Autodesk Inventor part; units mm, degrees
ref_plane "YZ Plane" through (0, 0, 0) normal (1, 0, 0) x (0, 1, 0)
ref_plane "XZ Plane" through (0, 0, 0) normal (0, 1, 0) x (-1, 0, 0)
ref_plane "XY Plane" through (0, 0, 0) normal (0, 0, 1) x (1, 0, 0)
sketch "Sketch1" plane through (0, 0, 0) normal (0, 0, 1) x (1, 0, 0)
  circle A0 centre (0, 0) radius 65
  dimension "d0" = 130
extrude "Extrusion1" add sketch "Sketch1" along normal blind 1.5
sketch "Sketch2" plane through (0, 0, 1.5) normal (0, 0, 1) x (1, 0, 0)
  circle A0 centre (0, 0) radius 57 construction
  point P0 (-57, 0)
  dimension "d3" = 114
hole "Hole1" at (-57, 0, 1.5) direction (0, 0, -1) diameter 7 end through all
pattern_circular "Circular Pattern1" count 8 over 360 about axis through (0, 0, -10) along (0, 0, 1) of "Hole1"
properties material "Rubber"
Part model, mm, in its own coordinate system. Give positions to 0.01 mm unless a question says otherwise; leave off trailing zeros. Order: outer loops, then holes, each group sorted by start corner. A loop starts at its lowest first (then second) coordinate and runs counter-clockwise, first axis right, second up. Notation, with made-up numbers: (61.25, 22.5) - (86.25, 22.5) arc R33 ccw to (86.25, 52.5) - close; hole circle Ø1 at (28.5, 88). An arc over 180 degrees is marked (long way). One line per question, with ' | ' between items.
1. Drill centre lines: probe 1 along X at (y, z) = (40, 1.35); probe 2 along X at (y, z) = (38, 0.35); probe 3 along Y at (x, z) = (37.5, 1.3). Where is each one in solid material? Low to high.
Filled in:
probe 1: -51.23 to -43.79, -36.82 to 36.82, 43.79 to 51.23 | probe 2: -52.74 to -42.94, -37.67 to 37.67, 42.94 to 52.74 | probe 3: -53.09 to -42.4, -38.21 to 38.21, 42.4 to 53.09
2. Band-saw the part on D-D on x = -57. List the corners of the cut face in (y, z).
Filled in:
outline: (-31.24, 0) - (-3.5, 0) - (-3.5, 1.5) - (-31.24, 1.5) - close; (3.5, 0) - (31.24, 0) - (31.24, 1.5) - (3.5, 1.5) - close
3. Drop a flat-ended pin along its axis: P1, Ø6.5, axis at x = 40.31, y = 40.31, coming from the -Z side. Give the stop position or say it passes through.
Filled in:
P1: through
4. Band-saw the part on A-A on x = 0. List the corners of the cut face in (y, z), then the cut area to 3 significant figures.
Filled in:
outline: (-65, 0) - (-60.5, 0) - (-60.5, 1.5) - (-65, 1.5) - close; (-53.5, 0) - (53.5, 0) - (53.5, 1.5) - (-53.5, 1.5) - close; (60.5, 0) - (65, 0) - (65, 1.5) - (60.5, 1.5) - close | area: 174 mm²
